```python
from build123d import *

# Parameters (mm, degrees)
BOSS_EXTRUDE1_DEPTH = 30
SKETCH2_W           = 2.275234404095272
SKETCH2_H           = 5.578757672765283
SKETCH2_H_2         = 5.578757672765278
SKETCH2_W_2         = 2.275234404095273
CUT_EXTRUDE1_DEPTH  = 5
SKETCH3_W           = 0.76212713524626
SKETCH3_H           = 5.066614641044968
SKETCH3_W_2         = 0.7621271352462609
SKETCH3_H_2         = 5.066614641044964
BOSS_EXTRUDE3_DEPTH = 5
CHAMFER2_SIZE       = 0.1
FILLET1_R           = 0.1
FILLET2_R           = 0.1
FILLET3_R           = 0.1
FILLET4_R           = 0.1
CUT_EXTRUDE2_DEPTH  = 5
BOSS_EXTRUDE4_DEPTH = 5
CUT_EXTRUDE3_START  = -15.000000000000002
CUT_EXTRUDE3_DEPTH  = 15.000000000000002
SKETCH7_W           = 4.440002623823602
SKETCH7_H           = 5.125420819496185
BOSS_EXTRUDE5_DEPTH = 0.4
SKETCH8_R           = 0.5886376526308733
BOSS_EXTRUDE6_DEPTH = 0.4
FILLET7_R           = 4
SKETCH10_R          = 0.5938831394244329
SKETCH10_R_2        = 0.5938831394244335
SKETCH10_R_3        = 0.5938831394244324
CUT_EXTRUDE4_DEPTH  = 0.4
FILLET8_R           = 4
BOSS_EXTRUDE7_DEPTH = 3
FILLET10_R          = 1


with BuildPart() as part:
    # Sketch1 → Boss-Extrude1 (new body)
    with BuildSketch(Plane.XY):
        with BuildLine():
            Line((-17.679491924311083, 3.18e-15), (17.6794919243111, 9.68e-15))
            ThreePointArc((17.6794919243111, 9.68e-15), (26.339745962155618, 5.000000000000008), (26.339745962155554, 15.000000000000124))
            Line((26.339745962155554, 15.000000000000124), (8.66025403784446, 45.621778264910596))
            ThreePointArc((8.66025403784446, 45.621778264910596), (6.34e-15, 50.621778264910716), (-8.660254037844458, 45.6217782649106))
            Line((-8.660254037844458, 45.6217782649106), (-26.339745962155547, 15.000000000000128))
            ThreePointArc((-26.339745962155547, 15.000000000000128), (-26.33974596215561, 5), (-17.679491924311083, 3.18e-15))
        make_face()
    extrude(amount=BOSS_EXTRUDE1_DEPTH)

    # Sketch2 → Cut-Extrude1 (cut)
    with BuildSketch(Plane(origin=(26.25000000000001, 15.155444566227686, 0), x_dir=(0, 0, -1), z_dir=(0.8660254037844386, 0.5000000000000001, 0))):
        with Locations((-6.771970321494826, 16.50011569419462)):
            Rectangle(SKETCH2_W, SKETCH2_H)
        with Locations((-6.771970321494791, 6.500115694194619)):
            Rectangle(SKETCH2_W, SKETCH2_H_2)
        with Locations((-6.771970321494861, 26.50011569419462)):
            Rectangle(SKETCH2_W_2, SKETCH2_H_2)
    extrude(amount=-CUT_EXTRUDE1_DEPTH, mode=Mode.SUBTRACT)

    # Sketch3 → Boss-Extrude3 (add)
    with BuildSketch(Plane(origin=(21.919872981077837, 12.655444566227697, 0), x_dir=(0, 0, -1), z_dir=(0.8660254037844385, 0.5000000000000003, 0))):
        with Locations((-6.16632950078614, 16.43387561929032)):
            Rectangle(SKETCH3_W, SKETCH3_H)
        with Locations((-6.166329500786105, 6.433875619290319)):
            Rectangle(SKETCH3_W_2, SKETCH3_H_2)
        with Locations((-6.166329500786173, 26.43387561929032)):
            Rectangle(SKETCH3_W_2, SKETCH3_H_2)
    extrude(amount=BOSS_EXTRUDE3_DEPTH)

    # Chamfer2
    chamfer2_edges = [part.edges().sort_by_distance(p)[0] for p in [
        (22.229568061632925, 17.119036951852106, 7.909587523542427),
        (20.064504552171826, 15.869036951852106, 6.771970321494791),
        (22.229568061632925, 17.119036951852106, 5.634353119447155),
        (22.9999421529027, 20.78470988493815, 7.909587523542427),
        (24.39463157109402, 18.369036951852106, 6.771970321494791),
        (22.9999421529027, 20.78470988493815, 5.634353119447155),
        (23.033062190354865, 20.727344297322453, 6.547393068409235),
        (24.29971585061611, 18.533435802156895, 6.166329500786105),
        (23.033062190354865, 20.727344297322453, 5.785265933162975),
        (21.766408530093624, 22.92125279248801, 6.166329500786105),
    ]]
    chamfer(chamfer2_edges, length=CHAMFER2_SIZE)

    # Fillet1
    fillet1_edges = [part.edges().sort_by_distance(p)[0] for p in [
        (19.299715850616106, 27.19368984000128, 6.16632950078614),
        (18.033062190354862, 29.387598335166835, 5.78526593316301),
        (16.76640853009362, 31.581506830332394, 6.16632950078614),
        (18.033062190354862, 29.387598335166835, 6.54739306840927),
    ]]
    fillet(fillet1_edges, radius=FILLET1_R)

    # Fillet2
    fillet2_edges = [part.edges().sort_by_distance(p)[0] for p in [
        (14.299715850616103, 35.853943877845666, 6.166329500786174),
        (13.03306219035486, 38.047852373011224, 5.785265933163044),
        (11.766408530093619, 40.241760868176776, 6.166329500786174),
        (13.03306219035486, 38.047852373011224, 6.547393068409304),
    ]]
    fillet(fillet2_edges, radius=FILLET2_R)

    # Fillet3
    fillet3_edges = [part.edges().sort_by_distance(p)[0] for p in [
        (19.394631571094017, 27.02929098969649, 6.771970321494826),
        (17.999942152902698, 29.444963922782534, 5.63435311944719),
        (16.605252734711378, 31.860636855868577, 6.771970321494826),
        (17.999942152902698, 29.444963922782534, 7.909587523542462),
    ]]
    fillet(fillet3_edges, radius=FILLET3_R)

    # Fillet4
    fillet4_edges = [part.edges().sort_by_distance(p)[0] for p in [
        (14.394631571094019, 35.68954502754087, 6.771970321494861),
        (12.999942152902698, 38.105217960626916, 5.634353119447224),
        (11.605252734711378, 40.52089089371296, 6.771970321494861),
        (12.999942152902698, 38.105217960626916, 7.909587523542497),
    ]]
    fillet(fillet4_edges, radius=FILLET4_R)

    # Sketch4 → Cut-Extrude2 (cut)
    with BuildSketch(Plane(origin=(26.25000000000001, 15.155444566227686, 0), x_dir=(0, 0, -1), z_dir=(0.8660254037844386, 0.5000000000000001, 0))):
        with BuildLine():
            Line((-3.8958432599542903, 3.970131617300865), (-3.8958432599542903, 8.204946525104617))
            ThreePointArc((-3.8958432599542903, 8.204946525104617), (-2.601063388610214, 9.499726396448693), (-1.306283517266138, 8.204946525104617))
            Line((-1.306283517266138, 8.204946525104617), (-1.306283517266138, 3.970131617300865))
            ThreePointArc((-1.306283517266138, 3.970131617300865), (-2.6010633886102146, 2.675351745956789), (-3.8958432599542903, 3.970131617300865))
        make_face()
    extrude(amount=-CUT_EXTRUDE2_DEPTH, mode=Mode.SUBTRACT)

    # Sketch5 → Boss-Extrude4 (add)
    with BuildSketch(Plane(origin=(21.919872981077813, 12.655444566227686, 0), x_dir=(0, 0, -1), z_dir=(0.8660254037844386, 0.5000000000000001, 0))):
        with BuildLine():
            Line((-3.0743032660907055, 3.583059523641907), (-3.0743032660907055, 8.465676524321175))
            ThreePointArc((-3.0743032660907055, 8.465676524321175), (-2.5777456783409036, 8.962234112070977), (-2.0811880905911018, 8.465676524321175))
            Line((-2.0811880905911018, 8.465676524321175), (-2.0811880905911018, 3.583059523641907))
            ThreePointArc((-2.0811880905911018, 3.583059523641907), (-2.5777456783409036, 3.0865019358921053), (-3.0743032660907055, 3.583059523641907))
        make_face()
    extrude(amount=BOSS_EXTRUDE4_DEPTH)

    # Sketch6 → Cut-Extrude3 (cut)
    with BuildSketch(Plane.XY.offset(30).offset(CUT_EXTRUDE3_START)):
        with BuildLine():
            Line((7.482900883826271, 7.11e-15), (-14.749507157804135, 35.07488248099315))
            Line((-14.749507157804127, 35.074882480993146), (-26.339745962155547, 15.000000000000131))
            ThreePointArc((-26.339745962155547, 15.000000000000128), (-26.339745962155618, 5.000000000000002), (-17.679491924311083, 1.78e-15))
            Line((-17.679491924311083, 3.18e-15), (7.482900883826272, 7.8e-15))
        make_face()
    extrude(amount=CUT_EXTRUDE3_DEPTH, mode=Mode.SUBTRACT)

    # Sketch7 → Boss-Extrude5 (add)
    with BuildSketch(Plane(origin=(5.338169454747117, 3.383628201109945, 0), x_dir=(0, 0, 1), z_dir=(-0.8446196510865366, -0.5353668321800086, 0))):
        with Locations((21.730667204522547, 17.27804822628798)):
            Rectangle(SKETCH7_W, SKETCH7_H)
    extrude(amount=BOSS_EXTRUDE5_DEPTH)

    # Sketch8 → Boss-Extrude6 (add)
    with BuildSketch(Plane(origin=(5.000321594312501, 3.169481468237942, 0), x_dir=(0, 0, 1), z_dir=(-0.8446196510865364, -0.5353668321800086, 0))):
        with Locations(Location((21.747310709322676, 17.2480877915433, 0), (0, 0, 90))):
            Circle(SKETCH8_R)
    extrude(amount=BOSS_EXTRUDE6_DEPTH)

    # Fillet7
    fillet7_edges = [part.edges().sort_by_distance(p)[0] for p in [
        (-3.633303136988933, 17.53744124049658, 14.999999999999998),
    ]]
    fillet(fillet7_edges, radius=FILLET7_R)

    # Sketch10 → Cut-Extrude4 (cut)
    with BuildSketch(Plane(origin=(26.25000000000001, 15.155444566227686, 0), x_dir=(0, 0, -1), z_dir=(0.8660254037844386, 0.5000000000000001, 0))):
        with Locations(Location((-23.062507434786994, 5.512963426255624, 0), (0, 0, 90))):
            Circle(SKETCH10_R)
        with Locations(Location((-21.062507434786994, 5.512963426255624, 0), (0, 0, 90))):
            Circle(SKETCH10_R)
        with Locations(Location((-21.062507434786998, 7.512963426255624, 0), (0, 0, 90))):
            Circle(SKETCH10_R)
        with Locations(Location((-21.062507434787005, 9.512963426255624, 0), (0, 0, 90))):
            Circle(SKETCH10_R)
        with Locations(Location((-21.062507434787012, 11.512963426255624, 0), (0, 0, 90))):
            Circle(SKETCH10_R)
        with Locations(Location((-21.06250743478702, 13.512963426255624, 0), (0, 0, 90))):
            Circle(SKETCH10_R)
        with Locations(Location((-21.062507434787026, 15.512963426255624, 0), (0, 0, 90))):
            Circle(SKETCH10_R)
        with Locations(Location((-21.062507434787033, 17.512963426255624, 0), (0, 0, 90))):
            Circle(SKETCH10_R_2)
        with Locations(Location((-21.06250743478704, 19.512963426255624, 0), (0, 0, 90))):
            Circle(SKETCH10_R_2)
        with Locations(Location((-21.062507434787047, 21.512963426255624, 0), (0, 0, 90))):
            Circle(SKETCH10_R_3)
        with Locations(Location((-21.062507434787054, 23.512963426255627, 0), (0, 0, 90))):
            Circle(SKETCH10_R_3)
        with Locations(Location((-21.06250743478706, 25.512963426255624, 0), (0, 0, 90))):
            Circle(SKETCH10_R_2)
        with Locations(Location((-21.06250743478707, 27.512963426255624, 0), (0, 0, 90))):
            Circle(SKETCH10_R_3)
        with Locations(Location((-21.062507434787076, 29.512963426255624, 0), (0, 0, 90))):
            Circle(SKETCH10_R_3)
        with Locations(Location((-21.062507434787083, 31.512963426255627, 0), (0, 0, 90))):
            Circle(SKETCH10_R_3)
        with Locations(Location((-23.062507434787, 7.512963426255624, 0), (0, 0, 90))):
            Circle(SKETCH10_R)
        with Locations(Location((-23.06250743478701, 9.512963426255624, 0), (0, 0, 90))):
            Circle(SKETCH10_R)
        with Locations(Location((-23.062507434787015, 11.512963426255624, 0), (0, 0, 90))):
            Circle(SKETCH10_R)
        with Locations(Location((-23.062507434787022, 13.512963426255624, 0), (0, 0, 90))):
            Circle(SKETCH10_R)
        with Locations(Location((-23.06250743478703, 15.512963426255624, 0), (0, 0, 90))):
            Circle(SKETCH10_R)
        with Locations(Location((-23.062507434787037, 17.512963426255624, 0), (0, 0, 90))):
            Circle(SKETCH10_R_2)
        with Locations(Location((-23.062507434787044, 19.512963426255624, 0), (0, 0, 90))):
            Circle(SKETCH10_R_2)
        with Locations(Location((-23.06250743478705, 21.512963426255624, 0), (0, 0, 90))):
            Circle(SKETCH10_R_3)
        with Locations(Location((-23.062507434787058, 23.512963426255627, 0), (0, 0, 90))):
            Circle(SKETCH10_R_3)
        with Locations(Location((-23.062507434787065, 25.512963426255624, 0), (0, 0, 90))):
            Circle(SKETCH10_R_2)
        with Locations(Location((-23.06250743478707, 27.512963426255624, 0), (0, 0, 90))):
            Circle(SKETCH10_R_3)
        with Locations(Location((-23.062507434787076, 29.512963426255624, 0), (0, 0, 90))):
            Circle(SKETCH10_R_3)
        with Locations(Location((-23.062507434787083, 31.512963426255627, 0), (0, 0, 90))):
            Circle(SKETCH10_R_3)
    extrude(amount=-CUT_EXTRUDE4_DEPTH, mode=Mode.SUBTRACT)

    # Fillet8
    fillet8_edges = [part.edges().sort_by_distance(p)[0] for p in [
        (-3.633303136988933, 17.53744124049658, 30),
    ]]
    fillet(fillet8_edges, radius=FILLET8_R)

    # Sketch11 → Boss-Extrude7 (add)
    with BuildSketch(Plane.XY.offset(14.999999999999998)):
        Polygon((-17.006968087908213, 31.16484545395118), (-18.366459113620724, 28.81013792498318), (0, 0), (2.747041382032401, 5e-16), align=None)
    extrude(amount=BOSS_EXTRUDE7_DEPTH)

    # Fillet10
    fillet10_edges = [part.edges().sort_by_distance(p)[0] for p in [
        (-18.366459113620724, 28.81013792498318, 16.5),
        (0, 0, 16.5),
        (-9.183229556810362, 14.40506896249159, 18),
    ]]
    fillet(fillet10_edges, radius=FILLET10_R)


solid = part.part
```
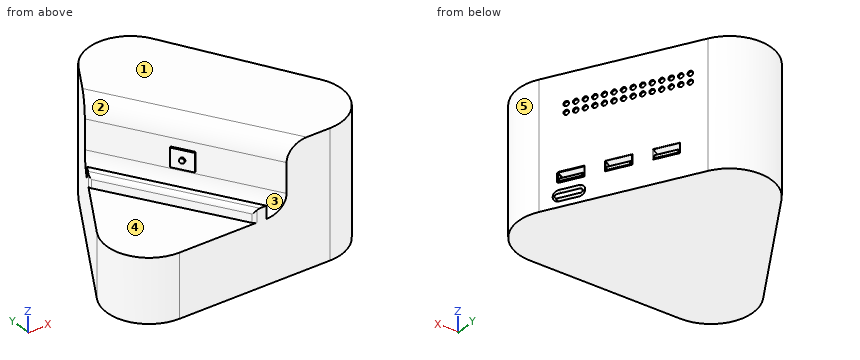
Source: CAD feature listing. Evaluate the final solid. Frame: model axes, mm. Face numbers are marked on the shaded views. A direction names the side the tool comes from. Give positions to 0.01 mm unless a question says otherwise; leave off trailing zeros. Loops run counter-clockwise (first coordinate to the right, second up) from the corner with the lowest first, then second, coordinate; pieces in that order, holes last. Notation, with made-up numbers: (31.25, -38) -> (73.25, -38) arc R20 cw to (73.25, 0) -> close; hole circle Ø1 at (-26, 10.5). An arc over 180 degrees is marked (long way). Use a Markdown table: item, result. Add a question column.
(1) Ray query, line 1 (Y direction, x = 12.5, z = 14); line 2 (Z direction, x = 22.5, y = 17); line 3 (X direction, y = 12, z = 15.5). Return the intervals inside material, ascending.
(2) First-contact query: pin 1 Ø6 at (y, z) = (36.5, 4.5) entering from +X; pin 2 Ø5 at (x, z) = (-19.5, 19.5) entering from -Y; pin 3 Ø2 at (x, y) = (16, 29) entering from -Z; pin 4 Ø12 at (x, z) = (-8, 19) entering from +Y. Flat tips, straight axial feed; report the tip coordinate or a pass-through.
(3) Section query B-B (x = -22). Output: boundary loops of the cut face in (y, z).
(4) Access query for the marked faces 4 and 5. Directions: +Z, -Z, +X, -X, +Y, -Y. A direction counts if a zero-diameter tool reaches every point of the face in a straight line with its end or side. Return the directions, or none.
(5) Section query A-A (z = 25.25). Output: boundary loops of the cut face in (x, y).
(6) Pull-direction query (Y, two-part tool) for the marked faces 1, 2 and 3; classes: +Y half, -Y half, draft (parallel to the pull), parting line (faces both ways), or undercut.
Checked values:
| question | item | result |
|---|---|---|
| 1 | line 1 | 0 to 38.97 |
| 1 | line 2 | 0 to 1.41, 2.09 to 3.06, 3.8 to 30 |
| 1 | line 3 | -7.65 to -4.86, -2.57 to 27.48 |
| 2 | pin 1 | x = 15.66 |
| 2 | pin 2 | y = 28.4 |
| 2 | pin 3 | z = 0 |
| 2 | pin 4 | y = 50.42 |
| 3 | outline | (0.98, 0) -> (22.52, 0) -> (22.52, 15) -> (0.98, 15) -> close |
| 4 | face 4 | +Z, -X, -Y |
| 4 | face 5 | +Z, -Z, +X |
| 5 | outline | (-14.75, 35.07) -> (7.48, 0) -> (17.68, 0) arc R10 ccw to (26.34, 15) -> (8.66, 45.62) arc R10 ccw to (-8.66, 45.62) -> close |
| 6 | face 1 | draft |
| 6 | face 2 | -Y half |
| 6 | face 3 | undercut |
